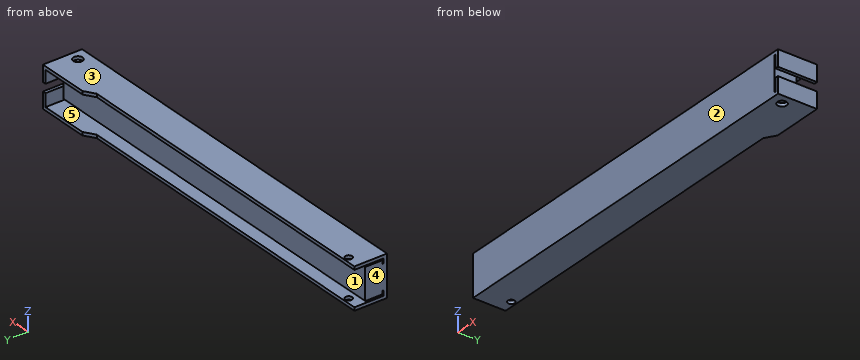
from build123d import *

# Parameters (mm, degrees)
SKETCH1_W           = 147.32
SKETCH1_H           = 15.24
BOSS_EXTRUDE1_DEPTH = 14.478
CUT_EXTRUDE2_DEPTH  = 146.1135
CUT_EXTRUDE5_REACH  = 78.601
SKETCH7_R           = 1.7145
SKETCH9_R           = 1.27
CUT_EXTRUDE6_DEPTH  = 77.60068984
CUT_EXTRUDE7_REACH  = 76.491
SKETCH11_W          = 0.381
SKETCH11_H          = 11.684
CUT_EXTRUDE8_REACH  = 77.233
SKETCH12_W          = 0.381
SKETCH12_H          = 0.676587602
CUT_EXTRUDE9_REACH  = 77.233
SKETCH13_W          = 0.381
SKETCH13_H          = 0.466412398
CUT_EXTRUDE10_REACH = 150.226
SKETCH14_W          = 1.6129
SKETCH14_H          = 14.478


with BuildPart() as part:
    # Sketch1 → Boss-Extrude1 (new body)
    with BuildSketch(Plane(origin=(0, 0, 0), x_dir=(1, 0, 0), z_dir=(0, 1, 0))):
        Rectangle(SKETCH1_W, SKETCH1_H)
    extrude(amount=BOSS_EXTRUDE1_DEPTH)

    # Sketch3 → Cut-Extrude2 (cut)
    with BuildSketch(Plane.ZY.offset(73.66)):
        Polygon((-6.4135, 14.478), (-6.4135, 13.2715), (-6.4135, 1.2065), (-4.466912398, 1.2065), (-4.466912398, 1.7145), (-5.736912398, 1.7145), (-5.736912398, 8.0645), (5.947087602, 8.0645), (5.947087602, 1.7145), (4.677087602, 1.7145), (4.677087602, 1.2065), (6.4135, 1.2065), (6.4135, 13.2715), (6.4135, 14.478), align=None)
    extrude(amount=-CUT_EXTRUDE2_DEPTH, mode=Mode.SUBTRACT)

    # Sketch7 → Cut-Extrude5 (cut, up to next)
    with BuildSketch(Plane.XY.offset(7.62), mode=Mode.PRIVATE) as cut_extrude5_sk1:
        Polygon((50.8, 12.074646248), (54.61, 14.478), (-73.66, 14.478), (-73.66, 12.074646248), align=None)
    cut_extrude5_tool1 = extrude(cut_extrude5_sk1.sketch, amount=-CUT_EXTRUDE5_REACH, mode=Mode.PRIVATE) & part.part
    # Sketch7 → Cut-Extrude5 (cut, up to next)
    with BuildSketch(Plane.XY.offset(7.62), mode=Mode.PRIVATE) as cut_extrude5_sk2:
        with Locations((69.85, 4.445)):
            Circle(SKETCH7_R)
    cut_extrude5_tool2 = extrude(cut_extrude5_sk2.sketch, amount=-CUT_EXTRUDE5_REACH, mode=Mode.PRIVATE) & part.part
    cut_extrude5_1 = cut_extrude5_tool1.solids().sort_by_distance((-10.472714, 13.282362, 7.62))[0]
    add(cut_extrude5_1, mode=Mode.SUBTRACT)
    cut_extrude5_2 = cut_extrude5_tool2.solids().sort_by_distance((69.85, 4.445, 7.62))[0]
    add(cut_extrude5_2, mode=Mode.SUBTRACT)
    cut_extrude5 = cut_extrude5_1 + cut_extrude5_2  # Cut-Extrude5 as one shape, for the pattern or mirror that repeats it

    # Sketch9 → Cut-Extrude6 (cut, through all)
    with BuildSketch(Plane.XY.offset(7.62)):
        with Locations((-68.58, 10.296646248)):
            Circle(SKETCH9_R)
    extrude(amount=-CUT_EXTRUDE6_DEPTH, mode=Mode.SUBTRACT)

    # Sketch11 → Cut-Extrude7 (cut, up to next)
    with BuildSketch(Plane(origin=(0, 8.0645, 0), x_dir=(1, 0, 0), z_dir=(0, 1, 0)), mode=Mode.PRIVATE) as cut_extrude7_sk1:
        with Locations((72.263, -0.105087602)):
            Rectangle(SKETCH11_W, SKETCH11_H)
    cut_extrude7_tool1 = extrude(cut_extrude7_sk1.sketch, amount=-CUT_EXTRUDE7_REACH, mode=Mode.PRIVATE) & part.part
    add(cut_extrude7_tool1.solids().sort_by_distance((72.263, 8.0645, 0.105088))[0], mode=Mode.SUBTRACT)

    # Sketch12 → Cut-Extrude8 (cut, up to next)
    with BuildSketch(Plane(origin=(0, 1.2065, 0), x_dir=(1, 0, 0), z_dir=(0, 1, 0)), mode=Mode.PRIVATE) as cut_extrude8_sk1:
        with Locations((72.263, 6.075206199)):
            Rectangle(SKETCH12_W, SKETCH12_H)
    cut_extrude8_tool1 = extrude(cut_extrude8_sk1.sketch, amount=-CUT_EXTRUDE8_REACH, mode=Mode.PRIVATE) & part.part
    add(cut_extrude8_tool1.solids().sort_by_distance((72.263, 1.2065, -6.075206))[0], mode=Mode.SUBTRACT)

    # Sketch13 → Cut-Extrude9 (cut, up to next)
    with BuildSketch(Plane(origin=(0, 1.2065, 0), x_dir=(1, 0, 0), z_dir=(0, 1, 0)), mode=Mode.PRIVATE) as cut_extrude9_sk1:
        with Locations((72.263, -6.180293801)):
            Rectangle(SKETCH13_W, SKETCH13_H)
    cut_extrude9_tool1 = extrude(cut_extrude9_sk1.sketch, amount=-CUT_EXTRUDE9_REACH, mode=Mode.PRIVATE) & part.part
    add(cut_extrude9_tool1.solids().sort_by_distance((72.263, 1.2065, 6.180294))[0], mode=Mode.SUBTRACT)

    # Sketch14 → Cut-Extrude10 (cut, up to next)
    with BuildSketch(Plane(origin=(73.66, 0, 0), x_dir=(0, 0, -1), z_dir=(1, 0, 0)), mode=Mode.PRIVATE) as cut_extrude10_sk1:
        with Locations((0.80645, 7.239)):
            Rectangle(SKETCH14_W, SKETCH14_H)
    cut_extrude10_tool1 = extrude(cut_extrude10_sk1.sketch, amount=-CUT_EXTRUDE10_REACH, mode=Mode.PRIVATE) & part.part
    # Sketch14 → Cut-Extrude10 (cut, up to next)
    with BuildSketch(Plane(origin=(73.66, 0, 0), x_dir=(0, 0, -1), z_dir=(1, 0, 0)), mode=Mode.PRIVATE) as cut_extrude10_sk2:
        with Locations((-0.80645, 7.239)):
            Rectangle(SKETCH14_W, SKETCH14_H)
    cut_extrude10_tool2 = extrude(cut_extrude10_sk2.sketch, amount=-CUT_EXTRUDE10_REACH, mode=Mode.PRIVATE) & part.part
    add(cut_extrude10_tool1.solids().sort_by_distance((73.66, 7.239, -0.80645))[0], mode=Mode.SUBTRACT)
    add(cut_extrude10_tool2.solids().sort_by_distance((73.66, 7.239, 0.80645))[0], mode=Mode.SUBTRACT)

    # Mirror1: Cut-Extrude5 across plane
    add(cut_extrude5.mirror(Plane(origin=(0, 0, 0), x_dir=(1, 0, 0), z_dir=(0, 0, -1))), mode=Mode.SUBTRACT)


solid = part.part
Verification items for the finished model (mm, model axes). Face numbers are marked on the shaded views. A direction names the side the tool comes from. Coordinates: 2 decimals unless noted, no trailing zeros. Write each loop counter-clockwise with the first axis right and the second up, starting at its lowest first coordinate (ties: lowest second). Pieces come first, ordered by that corner, then holes. Notation, with made-up numbers: (37.25, 50.25) -> (42.25, 50.25) arc R5 cw to (42.25, 57.25) -> close; hole circle Ø11 at (-10, 36.25). An arc over 180 degrees is marked (long way). One line per item, written item: value. Start each with the question number.
Q1. Thickness scan on L1, parallel to Z at x = -24, y = 3.25; L2, parallel to Y at x = 69.85, z = -6.75; L3, parallel to X at y = 4.75, z = 2.5. Record the ranges inside material, lowest first. Write a range as from..to.
Q2. Cross-section at B-B on x = -68.58. Enter the section's corners in (y, z).
Q3. Access from +Z, -Z, +X, -X, +Y, -Y to the whole of each face (thin tool, end or side, straight path). Record for the marked faces 4 and 5.
Q4. Cross-section at A-A on x = 69.85. Enter the section's corners in (y, z), and give its area (3 significant figures).
Q5. Go/stop test with flat-tipped pins: P1, Ø2.5, axis at x = 69.85, y = 4.445, coming from the -Z side; P2, Ø2, axis at x = -25.5, z = -5, coming from the +Y side. Record where each tip stops, or that it passes through.
Q6. Mould release check, pull along Z, two halves, no side actions. Record for the marked faces 1, 2 and 3: pulls with the +Z half, pulls with the -Z half, needs draft (parallel to the pull), parting line crosses it, or undercut.
Q7. Cross-section at C-C on x = 14. Enter the section's corners in (y, z), and give its area (3 significant figures).
Checked values:
1. L1: z = -7.62..-6.41, -5.74..5.95, 6.41..7.62
1. L2: y = 0..2.73, 6.16..14.48
1. L3: x = -73.66..72.07, 72.45..73.66
2. outline: (0, -7.62) -> (9.03, -7.62) -> (9.03, -6.41) -> (1.21, -6.41) -> (1.21, -4.47) -> (1.71, -4.47) -> (1.71, -5.74) -> (8.06, -5.74) -> (8.06, 5.95) -> (1.71, 5.95) -> (1.71, 4.68) -> (1.21, 4.68) -> (1.21, 6.41) -> (9.03, 6.41) -> (9.03, 7.62) -> (0, 7.62) -> close; (11.57, -7.62) -> (12.07, -7.62) -> (12.07, -6.41) -> (11.57, -6.41) -> close; (11.57, 6.41) -> (12.07, 6.41) -> (12.07, 7.62) -> (11.57, 7.62) -> close
3. face 4: +Z, -Z, -X, +Y, -Y
3. face 5: -X, +Y
4. outline: (0, -7.62) -> (2.73, -7.62) -> (2.73, -6.41) -> (1.21, -6.41) -> (1.21, -4.47) -> (1.71, -4.47) -> (1.71, -5.74) -> (8.06, -5.74) -> (8.06, 5.95) -> (1.71, 5.95) -> (1.71, 4.68) -> (1.21, 4.68) -> (1.21, 6.41) -> (2.73, 6.41) -> (2.73, 7.62) -> (0, 7.62) -> close; (6.16, -7.62) -> (14.48, -7.62) -> (14.48, -6.41) -> (6.16, -6.41) -> close; (6.16, 6.41) -> (14.48, 6.41) -> (14.48, 7.62) -> (6.16, 7.62) -> close
4. area: 121 mm²
5. P1: stops at z = -5.74
5. P2: stops at y = 8.06
6. face 1: undercut
6. face 2: needs draft
6. face 3: pulls with the +Z half
7. outline: (0, -7.62) -> (12.07, -7.62) -> (12.07, -6.41) -> (1.21, -6.41) -> (1.21, -4.47) -> (1.71, -4.47) -> (1.71, -5.74) -> (8.06, -5.74) -> (8.06, 5.95) -> (1.71, 5.95) -> (1.71, 4.68) -> (1.21, 4.68) -> (1.21, 6.41) -> (12.07, 6.41) -> (12.07, 7.62) -> (0, 7.62) -> close
7. area: 123 mm²
